Check sheet for the modelled part. Datum: model origin and axes. Units: mm. A direction names the side the tool comes from. Give positions to 0.01 mm unless a question says otherwise; leave off trailing zeros. Order: outer loops, then holes, each group sorted by start corner. A loop starts at its lowest first (then second) coordinate and runs counter-clockwise, first axis right, second up. Notation, with made-up numbers: M -23,49.25 L 35,49.25 A13 ccw 35,59.25 Z; hole C 25.25,-11 d11. An arc over 180 degrees is marked long. One line per question, with ' | ' between items. Start each with the question number.
```python
from build123d import *

# Parameters (mm, degrees)
F0_W     = 39.0892345458
F0_H     = 66.1229081452
F1_DEPTH = 0.762
F0_R     = 4.2603265816
F0_R_2   = 3.9515412254
F0_R_3   = 3.5979856565
F0_R_4   = 3.2023821092
F2_DEPTH = 6.096


# Not quite as in the source:
# - a feature of the source that left no trace in its solid (it failed there, or was rolled back) is left out


with BuildPart() as f1:
    # F0 (on Top) → F1 (new body)
    with BuildSketch(Plane.XY):
        with Locations((2.9225489125, -2.8168093413)):
            Rectangle(F0_W, F0_H)
    extrude(amount=F1_DEPTH)

    # F0 (on Top) → F2 (join)
    with BuildSketch(Plane.XY):
        Polygon((-20.7744576037, 15.3352888301), (-20.7744576037, 33.758495003), (-11.104892008, 33.758495003), (-31.6940061748, 93.3202803135), (-45.0146831572, 82.2209268808), align=None)
        with Locations((-33.4267839789, 83.2160338759)):
            Circle(F0_R, mode=Mode.SUBTRACT)
        Polygon((-11.104892008, 33.758495003), (-20.7744576037, 33.758495003), (-20.7744576037, 15.3352888301), (-20.7744576037, -30.4260663688), (-20.7744576037, -43.2014353573), (-10.0806253031, -43.2014353573), (20.0740266591, -43.2014353573), (26.9123706967, -43.2014353573), (26.9123706967, -30.5006168783), (26.9123706967, 16.304789111), (26.9123706967, 33.758495003), (13.8152288273, 33.758495003), align=None)
        with Locations((2.9225489125, -2.8168093413)):
            Rectangle(F0_W, F0_H, mode=Mode.SUBTRACT)
        Polygon((40.3667656029, 93.7842203212), (13.8152288273, 33.758495003), (26.9123706967, 33.758495003), (26.9123706967, 16.304789111), (61.2783841789, 83.0108523369), align=None)
        with Locations((44.0210402012, 84.6773162484)):
            Circle(F0_R_2, mode=Mode.SUBTRACT)
        Polygon((-20.7744576037, -43.2014353573), (-20.7744576037, -30.4260663688), (-59.1404661536, -69.1590458155), (-43.2117395103, -89.9672359228), (-10.0806253031, -43.2014353573), align=None)
        with Locations((-48.7702228129, -68.0264160037)):
            Circle(F0_R_3, mode=Mode.SUBTRACT)
        Polygon((59.6924833953, -76.2155726552), (26.9123706967, -30.5006168783), (26.9123706967, -43.2014353573), (20.0740266591, -43.2014353573), (41.1184616387, -97.2259193659), align=None)
        with Locations((52.4233952165, -76.2155726552)):
            Circle(F0_R_4, mode=Mode.SUBTRACT)
    extrude(amount=F2_DEPTH)


solid = f1.part
```
Item 1: Go/stop test with flat-tipped pins: P1, Ø1.5, axis at x = 44.5, z = 3.5, coming from the +Y side; P2, Ø1.8, axis at x = -4, z = 4.5, coming from the +Y side; P3, Ø1.6, axis at x = 4, z = 4, coming from the -Y side. Record where each tip stops, or that it passes through.
Item 2: Set-up check for faces 4 (the face through (30.45, -69.84, 3.01)), 5 (the face through (-39.69, -49.52, 3.01)), 6 (the face through (-16.622, -3, 3)), 7 (the face through (2, 33.758, 3)): record each of +Z, -Z, +X, -X, +Y, -Y from which the full face is reachable in a straight line by a thin tool's end or side.
Item 3: Draft check along Y on faces 1 (the face through (27.277, 64.192, 3.005)), 2 (the face through (5, -43.201, 3)), 3 (the face through (43.16, 80.82, 3.01)). Enter one of: released by +Y, released by -Y, zero draft, split by the parting line, or undercut.
Item 4: Section check A-A, the plane y = 65. Record the cut outline in (x, z), then the cut area to 3 significant figures.
Item 5: Section check C-C, the plane x = -27. Record the cut outline in (y, z).
Item 6: Scan lines: probe 1 along X at (y, z) = (-7.5, 1.5); probe 2 along Y at (x, z) = (0, 1.25); probe 3 along Y at (x, z) = (43, 5). Record each from-to range of solid material in increasing order. Write a range as [from, to].
Item 7: Section check B-B, the plane x = 52. Record the cut outline in (y, z).
Item 8: Section check D-D, the plane z = 4.75. Record the cut outline in (x, y), then the cut area to 3 significant figures.
Reported:
1) P1: stops at y = 92.04 | P2: stops at y = 33.76 | P3: stops at y = -43.2
2) face 4: +Z, -Z, -Y | face 5: +Z, -Z, -X | face 6: +Z | face 7: +Z, -Z, +Y
3) face 1: released by +Y | face 2: released by -Y | face 3: undercut
4) outline: M -38.77,0 L -21.9,0 L -21.9,6.1 L -38.77,6.1 Z; M 27.63,0 L 52,0 L 52,6.1 L 27.63,6.1 Z | area: 251 mm^2
5) outline: M -67.08,0 L -36.71,0 L -36.71,6.1 L -67.08,6.1 Z; M 32.51,0 L 79.74,0 L 79.74,6.1 L 32.51,6.1 Z
6) probe 1: x = [-20.77, -16.62], [22.47, 26.91] | probe 2: y = [-43.2, -35.88], [30.24, 33.76] | probe 3: y = [-95.1, -52.94], [47.53, 80.86], [88.49, 92.43]
7) outline: M -84.92,0 L -79.39,0 L -79.39,6.1 L -84.92,6.1 Z; M -73.04,0 L -65.49,0 L -65.49,6.1 L -73.04,6.1 Z; M 65,0 L 87.79,0 L 87.79,6.1 L 65,6.1 Z
8) outline: M -59.14,-69.16 L -43.21,-89.97 L -10.08,-43.2 L 20.07,-43.2 L 41.12,-97.23 L 59.69,-76.22 L 26.91,-30.5 L 26.91,16.3 L 61.28,83.01 L 40.37,93.78 L 13.82,33.76 L -11.1,33.76 L -31.69,93.32 L -45.01,82.22 L -20.77,15.34 L -20.77,-30.43 Z; hole C -48.77,-68.03 d7.2; hole C -33.43,83.22 d8.52; hole M -16.62,-35.88 L 22.47,-35.88 L 22.47,30.24 L -16.62,30.24 Z; hole C 44.02,84.68 d7.9; hole C 52.42,-76.22 d6.4 | area: 5,410 mm^2
